```python
from build123d import *

# Parameters (mm, degrees)
CHAMFER1_SIZE           = 10
CUT_EXTRUDE1_DEPTH      = 245.361412666
CUT_EXTRUDE1_DEPTH_BACK = 245.361412666
SKETCH2_R               = 6
HOLE1_D                 = 12
HOLE1_DEPTH             = 23
CHAMFER2_SIZE           = 2


with BuildPart() as part:
    # Sketch1 → Revolve1 (revolve)
    with BuildSketch(Plane.XY, mode=Mode.PRIVATE) as revolve1_sk:
        Polygon((0, 0), (19, 0), (19, 157), (32.5, 157), (32.5, 227), (11, 227), (11, 240), (0, 240), align=None)
    revolve(revolve1_sk.sketch.rotate(Axis((0, 240, 0), (0, -1, 0)), 180), axis=Axis((0, 240, 0), (0, -1, 0)))

    # Chamfer1
    chamfer1_edges = [part.edges().sort_by_distance(p)[0] for p in [
        (32.5, 227, 0),
        (32.5, 157, 0),
    ]]
    chamfer(chamfer1_edges, length=CHAMFER1_SIZE)

    # Sketch2 → Cut-Extrude1 (cut, two sides: drawn at the far end of the back side and taken through both)
    with BuildSketch(Plane.XY.offset(-CUT_EXTRUDE1_DEPTH_BACK)):
        with Locations((0, 192)):
            Circle(SKETCH2_R)
    extrude(amount=CUT_EXTRUDE1_DEPTH + CUT_EXTRUDE1_DEPTH_BACK, mode=Mode.SUBTRACT)

    # Hole1
    with Locations(Plane(origin=(0, 240, 0), x_dir=(1, 0, 0), z_dir=(0, 1, 0))):
        with Locations((0, 0)):
            Hole(HOLE1_D / 2, depth=HOLE1_DEPTH)

    # Chamfer2
    chamfer2_edges = [part.edges().sort_by_distance(p)[0] for p in [
        (19, 0, 0),
    ]]
    chamfer(chamfer2_edges, length=CHAMFER2_SIZE)


solid = part.part
```
Could you check a few things on this model? Use its own coordinates, in mm. A direction names the side the tool comes from. Give positions to 0.01 mm unless a question says otherwise; leave off trailing zeros. Loops run counter-clockwise (first coordinate to the right, second up) from the corner with the lowest first, then second, coordinate; pieces in that order, holes last. Notation, with made-up numbers: (53.25, 30.25) - (73.25, 30.25) arc R16 ccw to (73.25, 52.25) - close; hole circle Ø9 at (-38.75, 31). An arc over 180 degrees is marked (long way). Answer in a Markdown table with one row per item. Add a question column.
Q1. If we section it at B-B (z = 0): List the corners of the cut face in (x, y) for me, plus the area to 3 significant figures.
Q2. If we section it at D-D (y = 45): List the corners of the cut face in (x, z) for me.
Q3. Please list where these lines run through material, in increasing order: L1, parallel to Z at x = 0, y = 230; L2, parallel to Y at x = 0, z = 13; L3, parallel to Y at x = 0, z = 1. Write a range as from..to.
Q4. If we section it at C-C (y = 192): List the corners of the cut face in (x, z) for me, plus the area to 3 significant figures.
Q5. Which directions (+Z, -Z, +X, -X, +Y, -Y) give clear straight access to the entire face, cutting with the end or side of a thin tool? Please do faces 1 (the face through (-10, 227, -5)), 2 (the face through (0, 0, 0)), 3 (the face through (4.119, 80.585, 18.548)).
Q6. If we section it at A-A (x = 0): List the corners of the cut face in (y, z) for me.
Q7. For pin 1 (9.5 mm diameter, centred on x = 0, z = 0, fed in from +Y); pin 2 (8 mm diameter, centred on x = 4, z = 24, fed in from +Y); pin 3 (6 mm diameter, centred on x = 3, y = 48, fed in from +Z), each with a flat end and sliding along its axis, tell me the tip position at first contact or that it passes through.
Q8. We'd pull the mould along X, two halves only. Please class faces 4 (the face through (6, 228, 0)), 5 (the face through (2.38, 233.59, 10.74)), 6 (the face through (-5, 240, 5)), 7 (the face through (-1.301, 186.143, -0.455)): +X half, -X half, draft (parallel to the pull), parting line (faces both ways), or undercut.
The answers:
| question | item | result |
|---|---|---|
| 1 | outline | (-32.5, 167) - (-22.5, 157) - (-19, 157) - (-19, 2) - (-17, 0) - (17, 0) - (19, 2) - (19, 157) - (22.5, 157) - (32.5, 167) - (32.5, 217) - (22.5, 227) - (11, 227) - (11, 240) - (6, 240) - (6, 217) - (-6, 217) - (-6, 240) - (-11, 240) - (-11, 227) - (-22.5, 227) - (-32.5, 217) - close; hole circle Ø12 at (0, 192) |
| 1 | area | 10,200 mm^2 |
| 2 | outline | circle Ø38 at (0, 0) |
| 3 | L1 | z = -11..-6, 6..11 |
| 3 | L2 | y = 0..186, 198..227 |
| 3 | L3 | y = 0..186, 198..217 |
| 4 | outline | (-6, -31.94) - (-6, 31.94) arc R32.5 ccw to start; (6, -31.94) arc R32.5 ccw to (6, 31.94) - close |
| 4 | area | 2,540 mm^2 |
| 5 | face 1 | +Y |
| 5 | face 2 | +Z, -Z, +X, -X, -Y |
| 5 | face 3 | -Y |
| 6 | outline | (0, -17) - (2, -19) - (157, -19) - (157, -22.5) - (167, -32.5) - (186, -32.5) - (186, 32.5) - (167, 32.5) - (157, 22.5) - (157, 19) - (2, 19) - (0, 17) - close; (198, -32.5) - (217, -32.5) - (227, -22.5) - (227, -11) - (240, -11) - (240, -6) - (217, -6) - (217, 6) - (240, 6) - (240, 11) - (227, 11) - (227, 22.5) - (217, 32.5) - (198, 32.5) - close |
| 7 | pin 1 | stops at y = 217 |
| 7 | pin 2 | stops at y = 227 |
| 7 | pin 3 | stops at z = 19 |
| 8 | face 4 | undercut |
| 8 | face 5 | parting line |
| 8 | face 6 | draft |
| 8 | face 7 | undercut |
